Source: CAD feature listing. Evaluate the final solid. Frame: model axes, mm. A direction names the side the tool comes from. Give positions to 0.01 mm unless a question says otherwise; leave off trailing zeros. Write each loop counter-clockwise with the first axis right and the second up, starting at its lowest first coordinate (ties: lowest second). Pieces come first, ordered by that corner, then holes.
Autodesk Inventor part; units mm, degrees
ref_plane "Work Plane1" through (-238.4764, 94.082, 198.5771) normal (0, 1, 0) x (-1, 0, 0)
ref_plane "YZ Plane" through (0, 0, 0) normal (1, 0, 0) x (0, 1, 0)
ref_plane "XZ Plane" through (0, 0, 0) normal (0, 1, 0) x (-1, 0, 0)
ref_plane "Work Plane1" through (-238.4764, 94.082, 198.5771) normal (0, 1, 0) x (-1, 0, 0)
ref_plane "Work Plane2" through (-231.6014, 94.082, 198.5771) normal (0, 1, 0) x (1, 0, 0)
sketch "Sketch1" plane through (-231.6014, 94.082, 198.5771) normal (0, 1, 0) x (1, 0, 0)
  line L0 (-13.5, 2) -> (0, 2)
  line L1 (-13.5, 0) -> (-13.5, 2)
  line L2 (0, 0) -> (-13.5, 0)
  line L3 (0, 0) -> (0, 2)
  line L4 (-13.5, 0) -> (0, 0)
  line L5 (0, 0) -> (0, 13)
  line L6 (0, 13) -> (-13.5, 13)
  line L7 (-13.5, 13) -> (-13.5, 0)
  point P0 (231.6014, 198.5771)
  point P1 (0, 2)
  dimension "d0" = 13
extrude "Extrusion1" add sketch "Sketch1" along normal blind 2
ref_plane "Work Plane3" through (-238.3514, 112.082, 188.5771) normal (0, 1, 0) x (1, 0, 0)
sketch "Sketch2" plane through (-238.3514, 112.082, 188.5771) normal (0, 1, 0) x (1, 0, 0)
  line L0 (-10, 0) -> (10, 0)
  point P0 (238.3514, 188.5771)
sketch "Sketch3" plane through (-245.1014, 94.082, 187.5771) normal (0, 0, -1) x (-1, 0, 0)
  line L0 (-13.5, 0) -> (0, 0)
  line L1 (0, 0) -> (0, 18)
  line L2 (0, 18) -> (-13.5, 18)
  line L3 (-13.5, 18) -> (-13.5, 0)
edge flange "Flange1" height 18 angle 90 thickness 2 bend radius 2 thickness toward (0, 0, -1) relief tear relief width 2 relief depth 1 edges at (-238.3514, 96.082, 185.5771) wall of the first edge with corners at (-231.6014, 94.082, 187.5771) (-245.1014, 94.082, 187.5771) (-245.1014, 112.082, 187.5771) (-231.6014, 112.082, 187.5771)
bend "Bend1"
corner "Corner1"
sketch "Sketch4" plane through (-245.1014, 112.082, 187.5771) normal (0, 0, 1) x (1, 0, 0)
  circle A0 centre (6.75, -6) radius 2
  line L0 (13.5, 0) -> (0, 0)
  line L1 (6.75, 0) -> (6.75, -8.3247) construction
  point P0 (245.1014, -112.082)
  point P1 (6.75, -4)
  dimension "d14" = 4
  dimension "d15" = 4
extrude "Extrusion2" cut sketch "Sketch4" against normal through all
equation "\"d3\" = Thickness"
equation "\"d4\" = BendReliefWidth"
equation "\"d5\" = BendReliefDepth"
equation "\"d6\" = MinimumRemnant"
equation "\"d7\" = TransitionRadius"
equation "\"d10\" = BendRadius"
equation "\"d11\" = CornerReliefSize"
equation "\"d12\" = GapSize"
equation "\"d13\" = JacobiRadiusSize"
equation "\"BendRadius\" = Thickness"
equation "\"BendReliefWidth\" = Thickness"
equation "\"BendReliefDepth\" = 0.5 * Thickness"
equation "\"CornerReliefSize\" = 4 * Thickness"
equation "\"MinimumRemnant\" = 2 * Thickness"
equation "\"TransitionRadius\" = BendRadius"
equation "\"JacobiRadiusSize\" = BendRadius"
equation "\"GapSize\" = Thickness"
properties part number "BackWheelMountingPlate" material "Steel, Alloy"
1. Line query: L1, parallel to Y at x = -243.5, z = 189.5; L2, parallel to Z at x = -239.5, y = 110.5; L3, parallel to Z at x = -232, y = 95.75. Output: solid intervals per line, ascending.
2. Cut plane D-D, the plane y = 102.75. Return the cut outline in (x, z), then the cut area to 3 significant figures.
3. Mould query, pull axis Y, two halves, no side actions, for faces 1 (the flat face through (-245.101, 100, 187)), 2 (the cylindrical face through (-237.429, 104.308, 186.591)), 3 (the cylindrical face through (-238.45, 95.28, 186.72)). Classes: +Y half, -Y half, draft (parallel to the pull), parting line (faces both ways), or undercut.
4. Cut plane B-B, the plane z = 187.25. Return the cut outline in (x, y), then the cut area to 3 significant figures.
5. Access query for faces 4 (the flat face through (-238.4, 103.6, 185.577)), 5 (the flat face through (-238, 103, 187.577)). Directions: +Z, -Z, +X, -X, +Y, -Y. A direction counts if a zero-diameter tool reaches every point of the face in a straight line with its end or side. Return the directions, or none.
6. Cut plane C-C, the plane x = -235.5. Return the cut outline in (y, z).
7. Cut plane A-A, the plane x = -239.25. Return the cut outline in (y, z), then the cut area to 3 significant figures.
8. Contact query for flat-ended pins moving along their axis: P1, Ø2.5, axis at x = -237.5, z = 195, coming from the +Y side; P2, Ø3, axis at x = -238.35, y = 106.08, coming from the -Z side; P3, Ø1, axis at x = -233.5, y = 99.5, coming from the +Z side. Output: stop coordinate, or through.
Response values:
1. L1: y = 94.08 to 96.08
1. L2: z = 185.58 to 187.58
1. L3: z = 186.33 to 198.58
2. outline: (-245.1, 185.58) - (-231.6, 185.58) - (-231.6, 187.58) - (-245.1, 187.58) - close
2. area: 27.0 mm2
3. face 1: draft
3. face 2: undercut
3. face 3: -Y half
4. outline: (-245.1, 94.83) - (-231.6, 94.83) - (-231.6, 112.08) - (-245.1, 112.08) - close; hole circle Ø4 at (-238.35, 106.08)
4. area: 220 mm2
5. face 4: -Z, +X, -X, +Y, -Y
5. face 5: +Z, +X, -X, +Y
6. outline: (94.08, 189.58) arc R4 ccw to (98.08, 185.58) - (112.08, 185.58) - (112.08, 187.58) - (98.08, 187.58) arc R2 cw to (96.08, 189.58) - (96.08, 198.58) - (94.08, 198.58) - close
7. outline: (94.08, 189.58) arc R4 ccw to (98.08, 185.58) - (104.3, 185.58) - (104.3, 187.58) - (98.08, 187.58) arc R2 cw to (96.08, 189.58) - (96.08, 198.58) - (94.08, 198.58) - close; (107.87, 185.58) - (112.08, 185.58) - (112.08, 187.58) - (107.87, 187.58) - close
7. area: 48.3 mm2
8. P1: stops at y = 96.08
8. P2: passes through
8. P3: stops at z = 187.58
